```python
from build123d import *

# Parameters (mm, degrees)
SKETCH_1_R          = 75
EXTRUDE_1_DEPTH     = 3
SKETCH_2_R          = 17.5
SKETCH_2_R_2        = 25
CUT_EXTRUDE_1_DEPTH = 2
SKETCH_3_R          = 22.5
CUT_EXTRUDE_2_DEPTH = 2
SKETCH_12_R         = 17.5
CUT_EXTRUDE_7_DEPTH = 1
SKETCH_15_R         = 18.5
SKETCH_15_R_2       = 9
EXTRUDE_6_DEPTH     = 2.5
SKETCH_16_R         = 10
SKETCH_16_R_2       = 2.5
EXTRUDE_7_DEPTH     = 2.5
SKETCH_17_R         = 5
CUT_EXTRUDE_9_DEPTH = 1.5


with BuildPart() as part:
    # 草图1 → 凸台-拉伸1 (new body)
    with BuildSketch(Plane(origin=(0, 0, 0), x_dir=(1, 0, 0), z_dir=(0, 1, 0))):
        with Locations(Location((0, 0, 0), (0, 0, 270))):
            Circle(SKETCH_1_R)
    extrude(amount=EXTRUDE_1_DEPTH)

    # 草图2 → 切除-拉伸1 (cut)
    with BuildSketch(Plane(origin=(0, 3, 0), x_dir=(1, 0, 0), z_dir=(0, 1, 0))):
        with Locations(Location((-25, 0, 0), (0, 0, 270))):
            Circle(SKETCH_2_R)
        with Locations(Location((25, 0, 0), (0, 0, 270))):
            Circle(SKETCH_2_R_2)
    extrude(amount=-CUT_EXTRUDE_1_DEPTH, mode=Mode.SUBTRACT)

    # 草图3 → 切除-拉伸2 (cut)
    with BuildSketch(Plane.XZ):
        with Locations(Location((25, 0, 0), (0, 0, 270))):
            Circle(SKETCH_3_R)
    extrude(amount=-CUT_EXTRUDE_2_DEPTH, mode=Mode.SUBTRACT)

    # 草图12 → 切除-拉伸7 (cut)
    with BuildSketch(Plane(origin=(0, 1, 0), x_dir=(1, 0, 0), z_dir=(0, 1, 0))):
        with Locations(Location((-25, 0, 0), (0, 0, 270))):
            Circle(SKETCH_12_R)
    extrude(amount=-CUT_EXTRUDE_7_DEPTH, mode=Mode.SUBTRACT)

    # 草图15 → 凸台-拉伸6 (add)
    with BuildSketch(Plane.XZ):
        with Locations(Location((-25, 0, 0), (0, 0, 90))):
            Circle(SKETCH_15_R)
        with Locations(Location((-25, 0, 0), (0, 0, 270))):
            Circle(SKETCH_15_R_2, mode=Mode.SUBTRACT)
    extrude(amount=EXTRUDE_6_DEPTH)

    # 草图16 → 凸台-拉伸7 (add)
    with BuildSketch(Plane.XZ.offset(2.5)):
        with Locations(Location((-25, 0, 0), (0, 0, 270))):
            Circle(SKETCH_16_R)
        with Locations(Location((-25, 0, 0), (0, 0, 270))):
            Circle(SKETCH_16_R_2, mode=Mode.SUBTRACT)
    extrude(amount=EXTRUDE_7_DEPTH)

    # 草图17 → 切除-拉伸9 (cut)
    with BuildSketch(Plane(origin=(0, -2.5, 0), x_dir=(1, 0, 0), z_dir=(0, 1, 0))):
        with Locations(Location((-25, 0, 0), (0, 0, 270))):
            Circle(SKETCH_17_R)
    extrude(amount=-CUT_EXTRUDE_9_DEPTH, mode=Mode.SUBTRACT)


solid = part.part
```
Check sheet for the modelled part. Datum: model origin and axes. Units: mm. A direction names the side the tool comes from. Coordinates: 2 decimals unless noted, no trailing zeros. Order: outer loops, then holes, each group sorted by start corner. A loop starts at its lowest first (then second) coordinate and runs counter-clockwise, first axis right, second up. Notation, with made-up numbers: (65, 88.5) -> (90, 88.5) arc R38 cw to (90, 126.5) -> close; hole circle Ø8 at (-18, 2). An arc over 180 degrees is marked (long way). Write item = value, one per line. Start each with the question number.
1) Mould release check, pull along Z, two halves, no side actions. Record for faces 1 (the cylindrical face through (-17.914, -1.232, 17.089)), 2 (the flat face through (1, 3, 16)), 3 (the cylindrical face through (-22.52, -4.49, 0.33)): +Z half, -Z half, draft (parallel to the pull), parting line (faces both ways), or undercut.
2) Access from +Z, -Z, +X, -X, +Y, -Y to the whole of each face (thin tool, end or side, straight path). Record for faces 4 (the flat face through (28.82, 1, -22.34)), 5 (the cylindrical face through (-15.085, -3.732, 1.302)), 6 (the flat face through (-27, -5, -2)).
3) Cross-section at D-D (z = -40.5). Enter the section's corners in (x, y).
4) Material ranges on L1, parallel to X at y = 0.4, z = 0; L2, parallel to X at y = -4.15, z = 0; L3, parallel to X at y = -3.05, z = 0, recorded low to high.
5) Cross-section at A-A (x = -25). Enter the section's corners in (y, z).
6) Cross-section at C-C (x = -40). Enter the section's corners in (y, z).
7) Cross-section at B-B (z = 0). State how many separate pieces and enclosed holes the cut face has, then the cut area to 4 significant figures.
8) Go/stop test with flat-tipped pins: P1, Ø10, axis at x = 22, z = 22, coming from the -Y side; P2, Ø2, axis at x = -21, y = -2, coming from the -Z side; P3, Ø3, axis at x = -23, z = 0.5, coming from the +Y side; P4, Ø4.5, axis at x = -25, z = 0, coming from the +Y side. Record where each tip stops, or that it passes through.
Ans:
q1.face_1 = parting line
q1.face_2 = draft
q1.face_3 = undercut
q2.face_4 = +Y
q2.face_5 = -Y
q2.face_6 = +Z, -Z, +X, -X, -Y
q3.outline = (-63.12, 0) -> (63.12, 0) -> (63.12, 3) -> (-63.12, 3) -> close
q4.L1 = -75 to -42.5, -7.5 to 2.5, 47.5 to 75
q4.L2 = -35 to -27.5, -22.5 to -15
q4.L3 = -35 to -30, -20 to -15
q5.outline = (-5, -10) -> (-2.5, -10) -> (-2.5, -18.5) -> (0, -18.5) -> (0, -70.71) -> (3, -70.71) -> (3, -17.5) -> (0, -17.5) -> (0, -9) -> (-2.5, -9) -> (-2.5, -5) -> (-4, -5) -> (-4, -2.5) -> (-5, -2.5) -> close; (-5, 2.5) -> (-4, 2.5) -> (-4, 5) -> (-2.5, 5) -> (-2.5, 9) -> (0, 9) -> (0, 17.5) -> (3, 17.5) -> (3, 70.71) -> (0, 70.71) -> (0, 18.5) -> (-2.5, 18.5) -> (-2.5, 10) -> (-5, 10) -> close
q6.outline = (-2.5, -10.83) -> (0, -10.83) -> (0, -63.44) -> (3, -63.44) -> (3, -9.01) -> (0, -9.01) -> (0, 9.01) -> (3, 9.01) -> (3, 63.44) -> (0, 63.44) -> (0, 10.83) -> (-2.5, 10.83) -> close
q7.separate_pieces = 3
q7.enclosed_holes = 0
q7.area = 277.5 mm²
q8.P1 = 0
q8.P2 = -18.26
q8.P3 = -4
q8.P4 = through
